from build123d import *

# Parameters (mm, degrees)
F0_W     = 85
F0_H     = 200.8
F1_DEPTH = 12.7
F3_R     = 1.778
F4_DEPTH = 12.701
F5_R     = 1.778
F6_DEPTH = 12.701


with BuildPart() as f1:
    # F0 (on Front) → F1 (new body)
    with BuildSketch(Plane.XZ):
        Rectangle(F0_W, F0_H)
    extrude(amount=F1_DEPTH)

    # F3 (on face) → F4 (cut, through all)
    with BuildSketch(Plane.XZ.offset(12.7)):
        with Locations((-37.5, 56.3)):
            Circle(F3_R)
        with Locations((36.5, 32.3)):
            Circle(F3_R)
        with Locations((26.5, -81.7)):
            Circle(F3_R)
        with Locations((-37.5, -81.7)):
            Circle(F3_R)
    extrude(amount=-F4_DEPTH, mode=Mode.SUBTRACT)

    # F5 (on face) → F6 (cut, through all)
    with BuildSketch(Plane.XZ.offset(12.7)):
        Polygon((-28.519744, 56.3), (-37.5, 47.319744), (-37.5, -72.719744), (-28.519744, -81.7), (17.519744, -81.7), (23.869744, -75.35), (36.5, -75.35), (36.5, 23.319744), (30.15, 29.669744), (30.15, 56.3), align=None)
        with Locations((36.5, 32.3)):
            Circle(F5_R)
        with Locations((-37.5, -81.7)):
            Circle(F5_R)
        with Locations((26.5, -81.7)):
            Circle(F5_R)
    extrude(amount=-F6_DEPTH, mode=Mode.SUBTRACT)


solid = f1.part
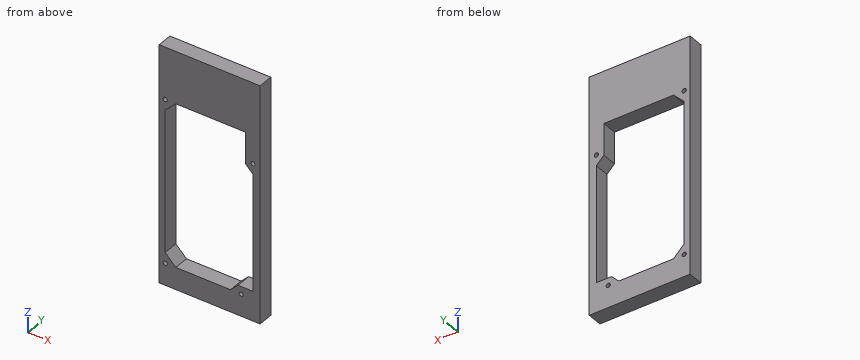
Read the model definition and answer for the solid it produces. Units are mm, in the model's axes. Coordinates: 2 decimals unless noted, no trailing zeros. Loops run counter-clockwise (first coordinate to the right, second up) from the corner with the lowest first, then second, coordinate; pieces in that order, holes last. Notation, with made-up numbers: (-13.75, 44.5) - (44.25, 44.5) arc R11 ccw to (44.25, 60.5) - close; hole circle Ø4 at (63.5, -36). An arc over 180 degrees is marked (long way). Answer in a Markdown table with one row per item.
Q1. Find section D-D on z = -30.5. Write down the section's boundary in (x, y).
Here are the results:
| item | result |
|---|---|
| outline | (-42.5, -12.7) - (-37.5, -12.7) - (-37.5, 0) - (-42.5, 0) - close; (36.5, -12.7) - (42.5, -12.7) - (42.5, 0) - (36.5, 0) - close |
Q2. Find section B-B on z = 32.3. Write down the section's boundary in (x, y).
Here are the results:
| item | result |
|---|---|
| outline | (-42.5, -12.7) - (-37.5, -12.7) - (-37.5, 0) - (-42.5, 0) - close; (30.15, -12.7) - (34.72, -12.7) - (34.72, 0) - (30.15, 0) - close; (38.28, -12.7) - (42.5, -12.7) - (42.5, 0) - (38.28, 0) - close |
Q3. Given P1, Ø2, axis at x = -15.5, z = 71, coming from the +Y side; P2, Ø12, axis at x = -29, z = -59.5, coming from the -Y side, each flat-ended and moving along its own axis, determine where each tip first touches the part or whether it passes through.
Here are the results:
| item | result |
|---|---|
| P1 | stops at y = 0 |
| P2 | passes through |
Q4. Straight lines are drawn through the part: line 1 along Z through (x, y) = (26.5, -9); line 2 along X through (y, z) = (-4.25, -82); line 3 along X through (y, z) = (-2.25, -5). For each, find the intervals that lie inside material, in ascending order. Write a range as [from, to].
Here are the results:
| item | result |
|---|---|
| line 1 | z = [-100.4, -83.48], [-79.92, -75.35], [56.3, 100.4] |
| line 2 | x = [-42.5, -39.25], [-35.75, 24.75], [28.25, 42.5] |
| line 3 | x = [-42.5, -37.5], [36.5, 42.5] |
Q5. Find section C-C on x = -16.5. Write down the section's boundary in (y, z).
Here are the results:
| item | result |
|---|---|
| outline | (-12.7, -100.4) - (0, -100.4) - (0, -81.7) - (-12.7, -81.7) - close; (-12.7, 56.3) - (0, 56.3) - (0, 100.4) - (-12.7, 100.4) - close |
Q6. Find section A-A on x = 26.5. Write down the section's boundary in (y, z), plus the area to 3 significant figures.
Here are the results:
| item | result |
|---|---|
| outline | (-12.7, -100.4) - (0, -100.4) - (0, -83.48) - (-12.7, -83.48) - close; (-12.7, -79.92) - (0, -79.92) - (0, -75.35) - (-12.7, -75.35) - close; (-12.7, 56.3) - (0, 56.3) - (0, 100.4) - (-12.7, 100.4) - close |
| area | 833 mm^2 |
